from build123d import *

# Parameters (mm, degrees)
ESQUISSE1_W        = 190
ESQUISSE1_H        = 90
BOSS_EXTRU_1_DEPTH = 4
CONG_1_R           = 55
CHANFREIN1_SIZE    = 25
CHANFREIN1_SIZE2   = 14.43375673


with BuildPart() as part:
    # Esquisse1 → Boss.-Extru.1 (new body)
    with BuildSketch(Plane(origin=(0, 0, 0), x_dir=(1, 0, 0), z_dir=(0, 1, 0))):
        Rectangle(ESQUISSE1_W, ESQUISSE1_H)
    extrude(amount=BOSS_EXTRU_1_DEPTH)

    # Congé1
    # the kernel refuses this fillet: 55 mm, written as the material it takes off along each edge
    with BuildSketch(Plane(origin=(-95, -137.5, 45), x_dir=(1, 0, 0), z_dir=(0, 1, 0))) as cong_1_piece_1:
        with BuildLine():
            CenterArc((CONG_1_R, CONG_1_R), CONG_1_R, 180, 90)
            Line((0, CONG_1_R), (0, 0))
            Line((0, 0), (CONG_1_R, 0))
        make_face()
    extrude(amount=279, mode=Mode.SUBTRACT)
    with BuildSketch(Plane(origin=(-95, -137.5, -45), x_dir=(1, 0, 0), z_dir=(0, 1, 0))) as cong_1_piece_2:
        with BuildLine():
            CenterArc((CONG_1_R, -CONG_1_R), CONG_1_R, 90, 90)
            Line((0, -CONG_1_R), (0, 0))
            Line((0, 0), (CONG_1_R, 0))
        make_face()
    extrude(amount=279, mode=Mode.SUBTRACT)

    # Chanfrein1
    chanfrein1_edges = [part.edges().sort_by_distance(p)[0] for p in [
        (95, 2, 45),
        (95, 2, -45),
    ]]
    chanfrein1_side = [part.faces().sort_by_distance(p)[0] for p in [
        (95, 2, 0),
    ]]
    chamfer(chanfrein1_edges, length=CHANFREIN1_SIZE, length2=CHANFREIN1_SIZE2, reference=chanfrein1_side[0])


solid = part.part
For this review, take the finished solid that the model builds, in its own axes (mm). Coordinates: 2 decimals unless noted, no trailing zeros. Order: outer loops, then holes, each group sorted by start corner. A loop starts at its lowest first (then second) coordinate and runs counter-clockwise, first axis right, second up. Notation, with made-up numbers: (-20, 17) - (8, 17) arc R29 cw to (8, 39) - close; hole circle Ø11 at (36.25, 1.25). An arc over 180 degrees is marked (long way). Answer as CSV lines item,"result". Start each with the question number.
1) To check wall thickness, follow line 1 along X through (y, z) = (3.6, -14); line 2 along X through (y, z) = (2.65, -35); line 3 along Z through (x, y) = (86.5, 0.8). State the ranges of each line that lie inside material, in increasing order. Write a range as [from, to].
2) Add section A-A (y = 3.05). State the section outline as (x, z) points, then the cut area to 3 significant figures.
3) Add section C-C (z = -22.5). State the section outline as (x, y) points, then the cut area to 3 significant figures.
4) Insertion check: P1, Ø12, axis at x = 64.5, z = -24.5, coming from the -Y side. The pin has a flat end and moves straight along its axis. Give the tip position at first contact, or say it passes through.
5) Add section B-B (z = -33.5). State the section outline as (x, y) points.
Result:
1,line 1,"[-89.49, 95]"
1,line 2,"[-71.62, 86.34]"
1,line 3,"[-34.72, 34.72]"
2,outline,"(-94.08, 0) arc R55 ccw to (-40, -45) - (80.57, -45) - (95, -20) - (95, 20) - (80.57, 45) - (-40, 45) arc R55 ccw to start"
2,area,"15,400 mm^2"
3,outline,"(-84.37, 0) - (93.56, 0) - (93.56, 4) - (-84.37, 4) - close"
3,area,"712 mm^2"
4,P1,"y = 0"
5,outline,"(-73.66, 0) - (87.21, 0) - (87.21, 4) - (-73.66, 4) - close"
